Verification items for this drawing (mm, ordinates from the low corner). A direction names the side the tool comes from. Round coordinates to 2 decimals unless told otherwise and drop trailing zeros. Write each loop counter-clockwise with the first axis right and the second up, starting at its lowest first coordinate (ties: lowest second). Pieces come first, ordered by that corner, then holes. Notation, with made-up numbers: M 50.5,-30.75 L 79.5,-30.75 A11 ccw 79.5,-22.75 Z; hole C -33,8.5 d5. An arc over 180 degrees is marked long. Write each question's results on one line, items separated by ' | '.
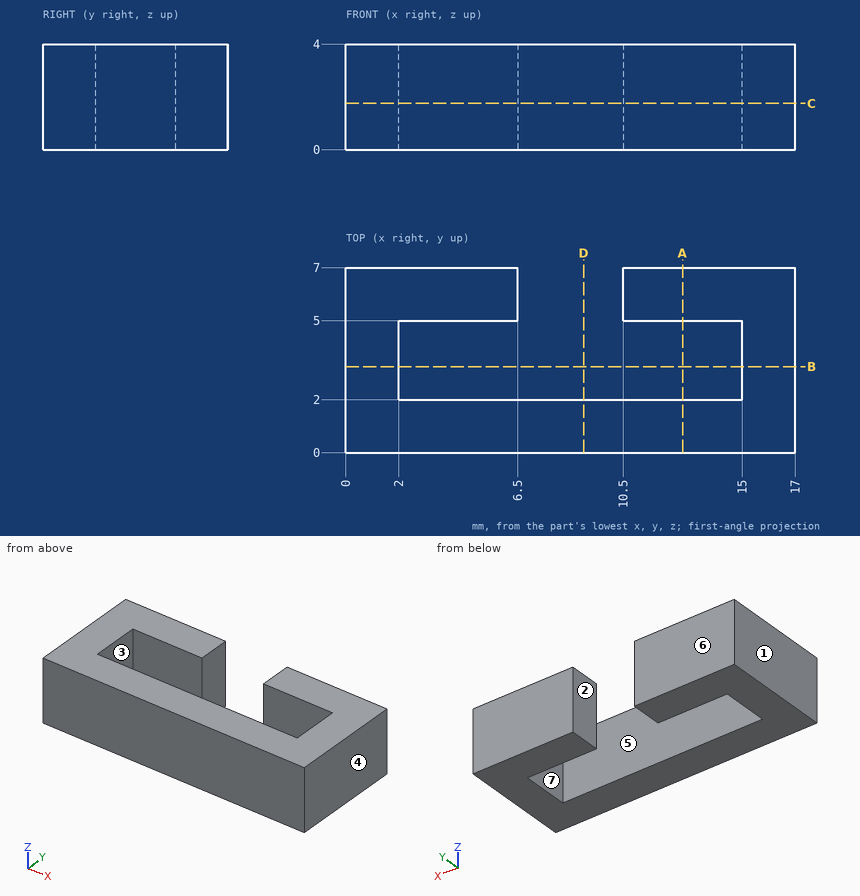
1) Access from +Z, -Z, +X, -X, +Y, -Y to the whole of each face (thin tool, end or side, straight path). Record for the marked faces 1, 2 and 3.
Calculated:
face 1: +Z, -Z, -X, +Y, -Y | face 2: +Z, -Z, +Y | face 3: +Z, -Z
2) Draft check along X on the marked faces 4, 5, 6 and 7. Enter one of: pulls with the +X half, pulls with the -X half, needs draft (parallel to the pull), parting line crosses it, or undercut.
Calculated:
face 4: pulls with the +X half | face 5: undercut | face 6: needs draft | face 7: undercut
3) Sectioned sample at A-A, the plane x = 12.75. Record the cut outline in (y, z), and give its area (3 significant figures).
Calculated:
outline: M 0,0 L 2,0 L 2,4 L 0,4 Z; M 5,0 L 7,0 L 7,4 L 5,4 Z | area: 16.0 mm²
4) Sectioned sample at B-B, the plane y = 3.25. Record the cut outline in (x, z).
Calculated:
outline: M 0,0 L 2,0 L 2,4 L 0,4 Z; M 15,0 L 17,0 L 17,4 L 15,4 Z
5) Sectioned sample at D-D, the plane x = 9. Record the cut outline in (y, z).
Calculated:
outline: M 0,0 L 2,0 L 2,4 L 0,4 Z
6) Material ranges on line 1 (Y direction, x = 12.5, z = 0.4); line 2 (X direction, y = 6.5, z = 0.8); line 3 (X direction, y = 3.5, z = 1.55), recorded low to high. Write a range as [from, to].
Calculated:
line 1: y = [0, 2], [5, 7] | line 2: x = [0, 6.5], [10.5, 17] | line 3: x = [0, 2], [15, 17]
7) Sectioned sample at C-C, the plane z = 1.75. Record the cut outline in (x, y), and give its area (3 significant figures).
Calculated:
outline: M 0,0 L 17,0 L 17,7 L 10.5,7 L 10.5,5 L 15,5 L 15,2 L 2,2 L 2,5 L 6.5,5 L 6.5,7 L 0,7 Z | area: 72.0 mm²
8) Depth check by flat-ended pin: P1, Ø0.9, axis at y = 3, z = 1.5, coming from the -X side. Enter the tip coordinate at first touch or a pass-through.
Calculated:
P1: stops at x = 0
